Verification items for the finished model (mm, model axes). Face numbers are marked on the shaded views. A direction names the side the tool comes from. Round coordinates to 2 decimals unless told otherwise and drop trailing zeros. Order: outer loops, then holes, each group sorted by start corner. A loop starts at its lowest first (then second) coordinate and runs counter-clockwise, first axis right, second up. Notation, with made-up numbers: (48.25, 89) -> (101.25, 89) arc R22 ccw to (101.25, 126) -> close; hole circle Ø3 at (73.25, 0). An arc over 180 degrees is marked (long way). Put each result on its own line as item: value.
from build123d import *

# Parameters (mm, degrees)
F0_W     = 39.405261
F0_H     = 14.46261
F0_R     = 9.525
F0_W_2   = 78.554068
F0_H_2   = 15.210686
F1_DEPTH = 25.4
F2_DEPTH = 37.592


with BuildPart() as f1:
    # F0 (on Top) → F1 (new body)
    with BuildSketch(Plane.XY):
        with Locations((-4.360169, 56.728363)):
            Rectangle(F0_W, F0_H)
        Polygon((15.342461, 49.497058), (-24.0628, 49.497058), (-24.0628, 0), (-63.211607, 0), (-63.211607, -53.48674), (15.342461, -53.48674), align=None)
        with Locations((-35.274969, -25.494586)):
            Circle(F0_R, mode=Mode.SUBTRACT)
        with Locations((-3.116944, 3.865009)):
            Circle(F0_R, mode=Mode.SUBTRACT)
        with Locations((-23.934573, -61.092083)):
            Rectangle(F0_W_2, F0_H_2)
    extrude(amount=F1_DEPTH)

    # F0 (on Top) → F2 (join)
    with BuildSketch(Plane.XY):
        with Locations((-4.360169, 56.728363)):
            Rectangle(F0_W, F0_H)
        with Locations((-23.934573, -61.092083)):
            Rectangle(F0_W_2, F0_H_2)
    extrude(amount=-F2_DEPTH)


solid = f1.part
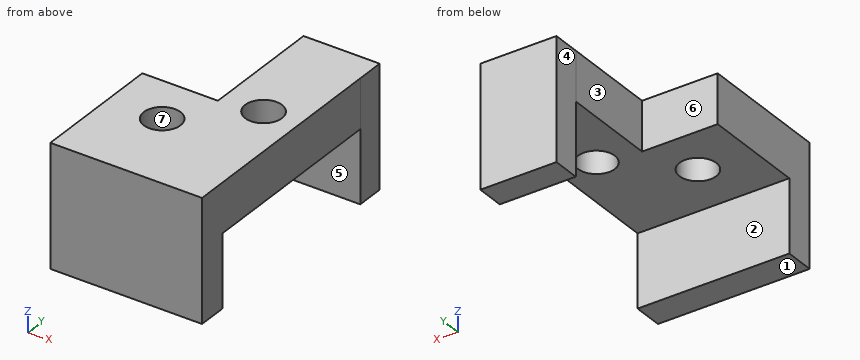
Item 1: Tool access check on the marked faces 1, 2 and 3. Record the directions out of +Z, -Z, +X, -X, +Y, -Y that give a thin tool (end or side, any length) a straight path to the whole face; none if there is none.
Check sheet entries:
face 1: -Z, +X, -X, +Y, -Y
face 2: -Z, +X, -X
face 3: +Z, -Z, -X, +Y
Item 2: Gauge pin test, flat ends, axial feed: pin 1 Ø4.5 at (y, z) = (58, 8.5) entering from -X; pin 2 Ø3 at (x, z) = (-45.5, -16.5) entering from +Y; pin 3 Ø6 at (x, z) = (-52, 7) entering from +Y. Record the tip position at first contact, or that the pin passes through.
Check sheet entries:
pin 1: stops at x = -24.06
pin 2: stops at y = -53.49
pin 3: stops at y = 0
Item 3: Section check C-C on x = -16. Record the boundary of the cut face in (y, z), then the cut area to 3 significant figures.
Check sheet entries:
outline: (-68.7, -37.59) -> (-53.49, -37.59) -> (-53.49, 0) -> (49.5, 0) -> (49.5, -37.59) -> (63.96, -37.59) -> (63.96, 25.4) -> (-68.7, 25.4) -> close
area: 4,480 mm^2
Item 4: Section check B-B on x = -39.5. Record the boundary of the cut face in (y, z), then the cut area to 3 significant figures.
Check sheet entries:
outline: (-68.7, -37.59) -> (-53.49, -37.59) -> (-53.49, 0) -> (-34.03, 0) -> (-34.03, 25.4) -> (-68.7, 25.4) -> close; (-16.96, 0) -> (0, 0) -> (0, 25.4) -> (-16.96, 25.4) -> close
area: 1,880 mm^2
Item 5: Release check for a two-part mould opening along Y. For the marked faces 4, 5, 6 and 7 record: +Y half, -Y half, draft (parallel to the pull), parting line (faces both ways), or undercut.
Check sheet entries:
face 4: draft
face 5: undercut
face 6: +Y half
face 7: undercut
Item 6: Material ranges on L1, parallel to X at y = 4.5, z = 15.5; L2, parallel to Y at x = 10, z = -11; L3, parallel to Z at x = -48, y = -8.5, recorded low to high. Write a range as [from, to].
Check sheet entries:
L1: x = [-24.06, -12.62], [6.39, 15.34]
L2: y = [-68.7, -53.49], [49.5, 63.96]
L3: z = [0, 25.4]
Item 7: Section check A-A on z = -21. Record the boundary of the cut face in (x, y), then the cut area to 3 significant figures.
Check sheet entries:
outline: (-63.21, -68.7) -> (15.34, -68.7) -> (15.34, -53.49) -> (-63.21, -53.49) -> close; (-24.06, 49.5) -> (15.34, 49.5) -> (15.34, 63.96) -> (-24.06, 63.96) -> close
area: 1,760 mm^2
Item 8: Section check D-D on y = -49. Record the boundary of the cut face in (x, z), then the cut area to 3 significant figures.
Check sheet entries:
outline: (-63.21, 0) -> (15.34, 0) -> (15.34, 25.4) -> (-63.21, 25.4) -> close
area: 2,000 mm^2
